Can you work these out from the model? Positions are in its coordinate system, mm. A direction names the side the tool comes from. Give positions to 0.01 mm unless a question says otherwise; leave off trailing zeros. Write each loop counter-clockwise with the first axis right and the second up, starting at its lowest first coordinate (ties: lowest second). Pieces come first, ordered by that corner, then holes. Notation, with made-up numbers: (-24, 43) -> (-12, 43) arc R10 cw to (-12, 56) -> close; hole circle Ø2 at (4, -31.75). An arc over 180 degrees is marked (long way). One line per item, written item: value.
from build123d import *

# Parameters (mm, degrees)
SKETCH1_W           = 50
SKETCH1_H           = 50
BOSS_EXTRUDE1_DEPTH = 3
SKETCH2_W           = 5
SKETCH2_H           = 3.320363524
SKETCH2_W_2         = 3.320363524
SKETCH2_H_2         = 5
CUT_EXTRUDE1_DEPTH  = 3
SKETCH4_W           = 3.2
SKETCH4_H           = 3
CUT_EXTRUDE2_DEPTH  = 12
SKETCH5_W           = 3
SKETCH5_H           = 3.2
CUT_EXTRUDE3_DEPTH  = 12
SKETCH6_W           = 3.2
SKETCH6_H           = 3
CUT_EXTRUDE4_DEPTH  = 12
SKETCH8_W           = 3
SKETCH8_H           = 3.2
CUT_EXTRUDE5_DEPTH  = 12
SKETCH9_W           = 6
SKETCH9_H           = 3
SKETCH9_W_2         = 3
SKETCH9_H_2         = 6
CUT_EXTRUDE6_DEPTH  = 12


with BuildPart() as part:
    # Sketch1 → Boss-Extrude1 (new body)
    with BuildSketch(Plane.XY):
        with Locations((3.733082315, -9.148044693)):
            Rectangle(SKETCH1_W, SKETCH1_H)
    extrude(amount=BOSS_EXTRUDE1_DEPTH)

    # Sketch2 → Cut-Extrude1 (cut)
    with BuildSketch(Plane.XY.offset(3)):
        with Locations((-11.266917685, 14.191773545)):
            Rectangle(SKETCH2_W, SKETCH2_H)
        with Locations((8.733082315, 14.191773545)):
            Rectangle(SKETCH2_W, SKETCH2_H)
        with Locations((-1.266917685, 14.191773545)):
            Rectangle(SKETCH2_W, SKETCH2_H)
        with Locations((18.733082315, 14.191773545)):
            Rectangle(SKETCH2_W, SKETCH2_H)
        with Locations((27.072900553, 5.851955307)):
            Rectangle(SKETCH2_W_2, SKETCH2_H_2)
        with Locations((27.072900553, -4.148044693)):
            Rectangle(SKETCH2_W_2, SKETCH2_H_2)
        with Locations((27.072900553, -14.148044693)):
            Rectangle(SKETCH2_W_2, SKETCH2_H_2)
        with Locations((27.072900553, -24.148044693)):
            Rectangle(SKETCH2_W_2, SKETCH2_H_2)
        with Locations((18.733082315, -32.487862931)):
            Rectangle(SKETCH2_W, SKETCH2_H)
        with Locations((8.733082315, -32.487862931)):
            Rectangle(SKETCH2_W, SKETCH2_H)
        with Locations((-1.266917685, -32.487862931)):
            Rectangle(SKETCH2_W, SKETCH2_H)
        with Locations((-11.266917685, -32.487862931)):
            Rectangle(SKETCH2_W, SKETCH2_H)
        with Locations((-19.606735923, -24.148044693)):
            Rectangle(SKETCH2_W_2, SKETCH2_H_2)
        with Locations((-19.606735923, -14.148044693)):
            Rectangle(SKETCH2_W_2, SKETCH2_H_2)
        with Locations((-19.606735923, -4.148044693)):
            Rectangle(SKETCH2_W_2, SKETCH2_H_2)
        with Locations((-19.606735923, 5.851955307)):
            Rectangle(SKETCH2_W_2, SKETCH2_H_2)
    extrude(amount=-CUT_EXTRUDE1_DEPTH, mode=Mode.SUBTRACT)

    # Sketch4 → Cut-Extrude2 (cut)
    with BuildSketch(Plane(origin=(0, 12.531591783, 0), x_dir=(1, 0, 0), z_dir=(0, 1, 0))):
        with Locations((-1.266917685, -1.5)):
            Rectangle(SKETCH4_W, SKETCH4_H)
        with Locations((8.733082315, -1.5)):
            Rectangle(SKETCH4_W, SKETCH4_H)
    extrude(amount=-CUT_EXTRUDE2_DEPTH, mode=Mode.SUBTRACT)

    # Sketch5 → Cut-Extrude3 (cut)
    with BuildSketch(Plane(origin=(25.412718791, 0, 0), x_dir=(0, 0, -1), z_dir=(1, 0, 0))):
        with Locations((-1.5, -4.148044693)):
            Rectangle(SKETCH5_W, SKETCH5_H)
        with Locations((-1.5, -14.148044693)):
            Rectangle(SKETCH5_W, SKETCH5_H)
    extrude(amount=-CUT_EXTRUDE3_DEPTH, mode=Mode.SUBTRACT)

    # Sketch6 → Cut-Extrude4 (cut)
    with BuildSketch(Plane.XZ.offset(30.827681169)):
        with Locations((-1.266917685, 1.5)):
            Rectangle(SKETCH6_W, SKETCH6_H)
        with Locations((8.733082315, 1.5)):
            Rectangle(SKETCH6_W, SKETCH6_H)
    extrude(amount=-CUT_EXTRUDE4_DEPTH, mode=Mode.SUBTRACT)

    # Sketch8 → Cut-Extrude5 (cut)
    with BuildSketch(Plane.ZY.offset(17.946554161)):
        with Locations((1.5, -14.148044693)):
            Rectangle(SKETCH8_W, SKETCH8_H)
        with Locations((1.5, -4.148044693)):
            Rectangle(SKETCH8_W, SKETCH8_H)
    extrude(amount=-CUT_EXTRUDE5_DEPTH, mode=Mode.SUBTRACT)

    # Sketch9 → Cut-Extrude6 (cut)
    with BuildSketch(Plane(origin=(0, 0, 0), x_dir=(-1, 0, 0), z_dir=(0, 0, -1))):
        with Locations((-8.733082315, -24.327681169)):
            Rectangle(SKETCH9_W, SKETCH9_H)
        with Locations((1.266917685, -24.327681169)):
            Rectangle(SKETCH9_W, SKETCH9_H)
        with Locations((-18.912718791, -4.148044693)):
            Rectangle(SKETCH9_W_2, SKETCH9_H_2)
        with Locations((-18.912718791, -14.148044693)):
            Rectangle(SKETCH9_W_2, SKETCH9_H_2)
        with Locations((1.266917685, 6.031591783)):
            Rectangle(SKETCH9_W, SKETCH9_H)
        with Locations((-8.733082315, 6.031591783)):
            Rectangle(SKETCH9_W, SKETCH9_H)
        with Locations((11.446554161, -14.148044693)):
            Rectangle(SKETCH9_W_2, SKETCH9_H_2)
        with Locations((11.446554161, -4.148044693)):
            Rectangle(SKETCH9_W_2, SKETCH9_H_2)
    extrude(amount=-CUT_EXTRUDE6_DEPTH, mode=Mode.SUBTRACT)


solid = part.part
1) If we section it at B-B (x = 19): Write out the boundary of the cut face in (y, z).
Answer list:
outline: (-30.83, 0) -> (-17.15, 0) -> (-17.15, 3) -> (-30.83, 3) -> close; (-11.15, 0) -> (-7.15, 0) -> (-7.15, 3) -> (-11.15, 3) -> close; (-1.15, 0) -> (12.53, 0) -> (12.53, 3) -> (-1.15, 3) -> close
2) I need wall thicknesses on L1, parallel to Y at x = 14, z = 2; L2, parallel to Y at x = -11, z = 2.6; L3, parallel to X at y = 7, z = 2.3. Which ranges of each line are inside material? Lowest first, please.
Answer list:
L1: y = -34.15 to -15.75, -12.55 to -5.75, -2.55 to 15.85
L2: y = -30.83 to -17.15, -11.15 to -7.15, -1.15 to 12.53
L3: x = -17.95 to -4.27, 1.73 to 5.73, 11.73 to 25.41
3) If we section it at A-A (y = 5.5): Write out the boundary of the cut face in (x, z).
Answer list:
outline: (-17.95, 0) -> (-4.27, 0) -> (-4.27, 3) -> (-17.95, 3) -> close; (1.73, 0) -> (5.73, 0) -> (5.73, 3) -> (1.73, 3) -> close; (11.73, 0) -> (25.41, 0) -> (25.41, 3) -> (11.73, 3) -> close
4) For faces 5 (the face through (-15, -15.748, 1)), 6 (the face through (3, -9, 0)), 7 (the face through (13.413, -4, 2)), 8 (the face through (6.233, 14, 2)), 9 (the face through (1.733, -24, 1)), which set-ups out of +Z, -Z, +X, -X, +Y, -Y let a thin tool reach every point of the face, with its end or its side?
Answer list:
face 5: +Z, -Z, -X
face 6: -Z, +X, -X, +Y, -Y
face 7: +Z, -Z, +X
face 8: +Z, -Z, +Y
face 9: +Z, -Z
5) We'd pull the mould along Y, two halves only. Please class faces 1 (the face through (-4, 7.532, 1)), 2 (the face through (28.733, 1, 1)), 3 (the face through (-20, -21.648, 2)), 4 (the face through (25, -34.148, 1)): released by +Y, released by -Y, zero draft, split by the parting line, or undercut.
Answer list:
face 1: undercut
face 2: zero draft
face 3: undercut
face 4: released by -Y
6) Will these pins go through, and if not, where does the flat tip stop? pin 1 (1.5 mm diameter, centred on x = -12, z = 1, fed in from +Y); pin 2 (1.5 mm diameter, centred on x = -1, z = 2, fed in from -Y).
Answer list:
pin 1: stops at y = 12.53
pin 2: stops at y = -18.83
